Read the model definition and answer for the solid it produces. Units are mm, in the model's axes. A direction names the side the tool comes from. Give positions to 0.01 mm unless a question says otherwise; leave off trailing zeros. Loops run counter-clockwise (first coordinate to the right, second up) from the corner with the lowest first, then second, coordinate; pieces in that order, holes last. Notation, with made-up numbers: (46, 17.25) - (97, 17.25) arc R23 ccw to (97, 47.25) - close; hole circle Ø2 at (4.25, 22). An arc over 180 degrees is marked (long way). Write each question's results on one line, items separated by ' | '. Start each with the question number.
Q1. Find the intervals of material crossed by line 1 (Y direction, x = 20, z = -6.5); line 2 (Y direction, x = -16, z = -8); line 3 (Y direction, x = 0, z = 4.5), in increasing order. Write a range as from..to.
Q2. The part is cut by section B-B, the plane x = 0. Write down the section's boundary in (y, z).
Q3. Given pin 1 (0.8 mm diameter, centred on y = 2.5, z = -3, fed in from +X); pin 2 (2 mm diameter, centred on x = 18.5, z = -5, fed in from -Y); pin 3 (5.5 mm diameter, centred on x = 11.5, z = -4.5, fed in from +Y), each flat-ended and moving along its own axis, determine where each tip first touches the part or whether it passes through.
Q4. The part is cut by section A-A, the plane z = -11. Write down the section's boundary in (x, y), plus the area to 3 significant figures.
Q5. The part is cut by section C-C, the plane y = 10. Write down the section's boundary in (x, z), plus the area to 3 significant figures.
Q6. Determine the mould class of faces 1 (the flat face through (-15, 32, 0)), 2 (the cylindrical face through (18.16, 31.69, -0.21)), 3 (the flat face through (27.5, 15.2, 0.2)) for opening direction Y: +Y half, -Y half, draft (parallel to the pull), parting line (faces both ways), or undercut.
Q7. For faces 4 (the flat face through (-19, 2, 0)), 5 (the cylindrical face through (-14.4, 27.57, 0.21)), 6 (the cylindrical face through (-21.84, 31.69, -0.21)), determine the directions among +Z, -Z, +X, -X, +Y, -Y from which every point of the face is accessible in a straight line to the end or side of a thin tool.
```python
from build123d import *

# Parameters (mm, degrees)
SKETCH1_R           = 2.5
BOSS_EXTRUDE1_DEPTH = 15


with BuildPart() as part:
    # Sketch1 → Boss-Extrude1 (new, symmetric)
    with BuildSketch(Plane.XY):
        with BuildLine():
            ThreePointArc((16.060946061, 4), (16.899910262, 3.800538423), (17.271733188, 3.022468012))
            Line((17.271733188, 3.022468012), (17.271733188, 2))
            Line((17.271733188, 2), (21.5, 2))
            ThreePointArc((21.5, 2), (22.207106781, 1.707106781), (22.5, 1))
            Line((22.5, 1), (22.5, 0))
            Line((22.5, 0), (30, 0))
            Line((30, 0), (24.933748499, 30.8112495))
            ThreePointArc((24.933748499, 30.8112495), (23.236027851, 33.811577593), (20, 35))
            Line((20, 35), (15, 35))
            Line((15, 35), (15, 29))
            Line((15, 29), (15, 27))
            Line((15, 27), (13, 27))
            Line((13, 27), (10, 27))
            ThreePointArc((10, 27), (0, 17), (-10, 27))
            Line((-10, 27), (-13, 27))
            ThreePointArc((-13, 27), (-14.414213562, 27.585786438), (-15, 29))
            Line((-15, 29), (-15, 35))
            Line((-15, 35), (-20, 35))
            ThreePointArc((-20, 35), (-23.236027851, 33.811577593), (-24.933748499, 30.8112495))
            Line((-24.933748499, 30.8112495), (-30, 0))
            Line((-30, 0), (-22.5, 0))
            Line((-22.5, 0), (-22.5, 1))
            ThreePointArc((-22.5, 1), (-22.207106781, 1.707106781), (-21.5, 2))
            Line((-21.5, 2), (-17.271733188, 2))
            Line((-17.271733188, 2), (-17.271733188, 3.022468012))
            ThreePointArc((-17.271733188, 3.022468012), (-16.899910262, 3.800538423), (-16.060946061, 4))
            Line((-16.060946061, 4), (16.060946061, 4))
        make_face()
        with Locations((-20, 30)):
            Circle(SKETCH1_R, mode=Mode.SUBTRACT)
        with Locations((20, 30)):
            Circle(SKETCH1_R, mode=Mode.SUBTRACT)
    extrude(amount=BOSS_EXTRUDE1_DEPTH, both=True)


solid = part.part
```
Check sheet entries:
1) line 1: y = 2..27.5, 32.5..35 | line 2: y = 4..35 | line 3: y = 4..17
2) outline: (4, -15) - (17, -15) - (17, 15) - (4, 15) - close
3) pin 1: stops at x = 29.65 | pin 2: stops at y = 2 | pin 3: stops at y = 27
4) outline: (-30, 0) - (-22.5, 0) - (-22.5, 1) arc R1 cw to (-21.5, 2) - (-17.27, 2) - (-17.27, 3.02) arc R1 cw to (-16.06, 4) - (16.06, 4) arc R1 cw to (17.27, 3.02) - (17.27, 2) - (21.5, 2) arc R1 cw to (22.5, 1) - (22.5, 0) - (30, 0) - (24.93, 30.81) arc R5 ccw to (20, 35) - (15, 35) - (15, 27) - (10, 27) arc R10 cw to (-10, 27) - (-13, 27) arc R2 cw to (-15, 29) - (-15, 35) - (-20, 35) arc R5 ccw to (-24.93, 30.81) - close; hole circle Ø5 at (-20, 30); hole circle Ø5 at (20, 30) | area: 1,300 mm^2
5) outline: (-28.36, -15) - (28.36, -15) - (28.36, 15) - (-28.36, 15) - close | area: 1,700 mm^2
6) face 1: draft | face 2: undercut | face 3: +Y half
7) face 4: +Z, -Z, -Y | face 5: +Z, -Z, +Y | face 6: +Z, -Z
